Work out the finished part from the listing and answer in its coordinate system (mm). A direction names the side the tool comes from. Coordinates: 2 decimals unless noted, no trailing zeros. Write each loop counter-clockwise with the first axis right and the second up, starting at its lowest first coordinate (ties: lowest second). Pieces come first, ordered by that corner, then holes. Notation, with made-up numbers: (18.25, 22.25) - (60.25, 22.25) arc R14 ccw to (60.25, 39.25) - close; hole circle Ø11 at (19.5, 5.5). An arc over 180 degrees is marked (long way). One line per item, written item: value.
Autodesk Inventor part; units mm, degrees
ref_plane "YZ Plane" through (0, 0, 0) normal (1, 0, 0) x (0, 1, 0)
ref_plane "XZ Plane" through (0, 0, 0) normal (0, 1, 0) x (-1, 0, 0)
ref_plane "XY Plane" through (0, 0, 0) normal (0, 0, 1) x (1, 0, 0)
sketch "Sketch1" plane through (0, 0, 0) normal (0, 0, 1) x (1, 0, 0)
  point P0 (0, 0)
sketch "Sketch2" plane through (0, 0, 0) normal (0, 0, 1) x (1, 0, 0)
  line L0 (-450, -125) -> (450, -125)
  line L1 (450, -125) -> (450, 125)
  line L2 (450, 125) -> (-450, 125)
  line L3 (-450, 125) -> (-450, -125)
  line L4 (-450, -125) -> (450, 125) construction
  line L5 (450, -125) -> (-450, 125) construction
  point P0 (0, 0)
  dimension "d0" = 900
  dimension "d1" = 250
extrude "Plate1" add sketch "Sketch2" along normal blind 3.048
sketch "Sketch3" plane through (450, 121.952, 3.048) normal (0, 1, 0) x (-1, 0, 0)
  line L0 (900, 0) -> (0, 0)
  line L1 (0, 0) -> (0, -25)
  line L2 (0, -25) -> (900, -25)
  line L3 (900, -25) -> (900, 0)
edge flange "Flange1" height 25 angle 90 thickness 3.048 bend radius 3.048 thickness toward (0, 1, 0) relief tear relief width 3.048 relief depth 1.524 corner gap 3.048 corner form 2 edges at (0, 125, 0) (0, -125, 0) (-450, 0, 0) (450, 0, 0) wall of the first edge with corners at (-450, 121.952, 3.048) (450, 121.952, 3.048) (450, 121.952, -21.952) (-450, 121.952, -21.952)
bend "Bend1"
corner "Corner1"
equation "\"d2\" = Thickness"
equation "\"d3\" = BendReliefWidth"
equation "\"d4\" = BendReliefDepth"
equation "\"d5\" = MinimumRemnant"
equation "\"d6\" = TransitionRadius"
equation "\"d9\" = BendRadius"
equation "\"d10\" = CornerReliefSize"
equation "\"d11\" = GapSize"
equation "\"d12\" = JacobiRadiusSize"
equation "\"BendRadius\" = Thickness"
equation "\"BendReliefWidth\" = Thickness"
equation "\"BendReliefDepth\" = 0.5 * Thickness"
equation "\"CornerReliefSize\" = 4 * Thickness"
equation "\"MinimumRemnant\" = 2 * Thickness"
equation "\"TransitionRadius\" = BendRadius"
equation "\"JacobiRadiusSize\" = BendRadius"
equation "\"GapSize\" = Thickness"
equation "\"Space5\" = 0"
equation "\"Space6\" = 0"
equation "\"Space7\" = 0"
properties part number "TapaUp"
Item 1: Given pin 1 (6.5 mm diameter, centred on x = -448, z = -1.5, fed in from +Y); pin 2 (5 mm diameter, centred on y = -120.5, z = -1.5, fed in from +X); pin 3 (3 mm diameter, centred on y = 122, z = 0, fed in from -X); pin 4 (5 mm diameter, centred on x = -447, z = -0.5, fed in from -Y), each flat-ended and moving along its own axis, determine where each tip first touches the part or whether it passes through.
Evaluation:
pin 1: stops at y = 119.8
pin 2: stops at x = 450
pin 3: stops at x = -443.9
pin 4: stops at y = -118.9
Item 2: Consider probe 1 along X at (y, z) = (-76, -13.5); probe 2 along Y at (x, z) = (-129, -17.75); probe 3 along Z at (x, y) = (-365, -16.5). Determine where each line is inside the solid, lowest interval first.
Evaluation:
probe 1: x = -450 to -446.95, 446.95 to 450
probe 2: y = -125 to -121.95, 121.95 to 125
probe 3: z = 0 to 3.05
Item 3: Section A-A, the plane z = -12.75 is taken. Determine the outline of the cut face in (x, y).
Evaluation:
outline: (-450, -119.8) - (-446.95, -119.8) - (-446.95, 119.8) - (-450, 119.8) - close; (-444.8, -125) - (444.8, -125) - (444.8, -121.95) - (-444.8, -121.95) - close; (-444.8, 121.95) - (444.8, 121.95) - (444.8, 125) - (-444.8, 125) - close; (446.95, -119.8) - (450, -119.8) - (450, 119.8) - (446.95, 119.8) - close
Item 4: Determine the mould class of faces 1 (the face through (450, -2, -13)), 2 (the face through (6, 125, -13)), 3 (the face through (6, 121.952, -12)) for opening direction Y: +Y half, -Y half, draft (parallel to the pull), parting line (faces both ways), or undercut.
Evaluation:
face 1: draft
face 2: +Y half
face 3: undercut
Item 5: Which of the six approach directions +Z, -Z, +X, -X, +Y, -Y give full straight-line access (tool end or side, diameter ignored) to faces 4 (the face through (-6, 2, 3.048)), 5 (the face through (-450, 2, -13)), 6 (the face through (-6, -121.952, -12)), 7 (the face through (-446.952, 2, -12)), 8 (the face through (-6, 2, 0))?
Evaluation:
face 4: +Z, +X, -X, +Y, -Y
face 5: +Z, -Z, -X, +Y, -Y
face 6: -Z, +X, -X
face 7: -Z, +Y, -Y
face 8: -Z
Item 6: Section C-C, the plane y = 104 is taken. Determine the outline of the cut face in (x, z).
Evaluation:
outline: (-450, -21.95) - (-446.95, -21.95) - (-446.95, -3.05) arc R3.05 cw to (-443.9, 0) - (443.9, 0) arc R3.05 cw to (446.95, -3.05) - (446.95, -21.95) - (450, -21.95) - (450, -3.05) arc R6.1 ccw to (443.9, 3.05) - (-443.9, 3.05) arc R6.1 ccw to (-450, -3.05) - close
Item 7: Section B-B, the plane x = 364 is taken. Determine the outline of the cut face in (y, z).
Evaluation:
outline: (-125, -21.95) - (-121.95, -21.95) - (-121.95, -3.05) arc R3.05 cw to (-118.9, 0) - (118.9, 0) arc R3.05 cw to (121.95, -3.05) - (121.95, -21.95) - (125, -21.95) - (125, -3.05) arc R6.1 ccw to (118.9, 3.05) - (-118.9, 3.05) arc R6.1 ccw to (-125, -3.05) - close
